Verification items for the finished model (mm, model axes). Face numbers are marked on the shaded views. A direction names the side the tool comes from. Coordinates: 2 decimals unless noted, no trailing zeros. Order: outer loops, then holes, each group sorted by start corner. A loop starts at its lowest first (then second) coordinate and runs counter-clockwise, first axis right, second up. Notation, with made-up numbers: M 83,7.5 L 134,7.5 A22 ccw 134,46.5 Z; hole C 63.5,-35.5 d11. An arc over 180 degrees is marked long. Return JSON: item names as keys, results as strings.
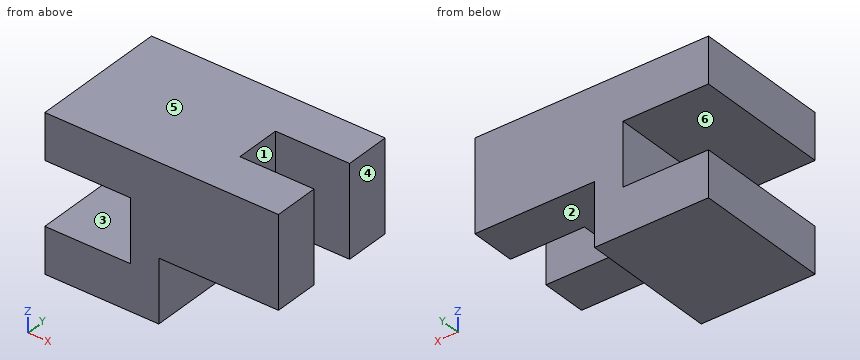
```python
from build123d import *

# Parameters (mm, degrees)
EXTRUDE_1_DEPTH     = 12
SKETCH_2_W          = 13
SKETCH_2_H          = 8
CUT_EXTRUDE_1_DEPTH = 24


with BuildPart() as part:
    # 草图1 → 凸台-拉伸1 (new, symmetric)
    with BuildSketch(Plane(origin=(0, 0, 0), x_dir=(1, 0, 0), z_dir=(0, 1, 0))):
        Polygon((0, 11), (0, 0), (-15, 0), (-15, -8), (26, -8), (26, 8), (5, 8), (5, 19), (-15, 19), (-15, 11), align=None)
    extrude(amount=EXTRUDE_1_DEPTH, both=True)

    # 草图2 → 切除-拉伸1 (cut)
    with BuildSketch(Plane.XY.offset(8)):
        with Locations((19.5, 0)):
            Rectangle(SKETCH_2_W, SKETCH_2_H)
    extrude(amount=-CUT_EXTRUDE_1_DEPTH, mode=Mode.SUBTRACT)


solid = part.part
```
Q1. Material ranges on line 1 along Z through (x, y) = (-5.5, 3.25); line 2 along X through (y, z) = (5.75, -2); line 3 along Y through (x, z) = (19.5, -0.5), recorded low to high.
Values:
{"line 1": "-19 to -11, 0 to 8", "line 2": "0 to 26", "line 3": "-12 to -4, 4 to 12"}
Q2. Cross-section at A-A, the plane x = 21. Record the boundary of the cut face in (y, z), and give its area (3 significant figures).
Values:
{"outline": "M -12,-8 L -4,-8 L -4,8 L -12,8 Z; M 4,-8 L 12,-8 L 12,8 L 4,8 Z", "area": "256 mm^2"}
Q3. Cross-section at D-D, the plane x = 5.5. Record the boundary of the cut face in (y, z).
Values:
{"outline": "M -12,-8 L 12,-8 L 12,8 L -12,8 Z"}
Q4. Tool access check on the marked faces 1, 2 and 3. Record the directions out of +Z, -Z, +X, -X, +Y, -Y that give a thin tool (end or side, any length) a straight path to the whole face; none if there is none.
Values:
{"face 1": "+Z, -Z, +X", "face 2": "-Z, +X, +Y, -Y", "face 3": "-X, +Y, -Y"}
Q5. Draft check along Z on the marked faces 4, 5 and 6. Enter one of: pulls with the +Z half, pulls with the -Z half, needs draft (parallel to the pull), parting line crosses it, or undercut.
Values:
{"face 4": "needs draft", "face 5": "pulls with the +Z half", "face 6": "undercut"}
Q6. Cross-section at B-B, the plane y = 2. Record the boundary of the cut face in (x, z).
Values:
{"outline": "M -15,-19 L 5,-19 L 5,-8 L 13,-8 L 13,8 L -15,8 L -15,0 L 0,0 L 0,-11 L -15,-11 Z"}
Q7. Go/stop test with flat-tipped pins: pin 1 (4 mm diameter, centred on y = -0.5, z = 0, fed in from +X); pin 2 (12 mm diameter, centred on y = -3, z = -15.5, fed in from +X); pin 3 (2 mm diameter, centred on x = 20.5, y = 4.5, fed in from -Z). Record where each tip stops, or that it passes through.
Values:
{"pin 1": "x = 13", "pin 2": "x = 5", "pin 3": "z = -8"}
Q8. Cross-section at C-C, the plane z = 5.25. Record the boundary of the cut face in (x, y), and give its area (3 significant figures).
Values:
{"outline": "M -15,-12 L 26,-12 L 26,-4 L 13,-4 L 13,4 L 26,4 L 26,12 L -15,12 Z", "area": "880 mm^2"}
